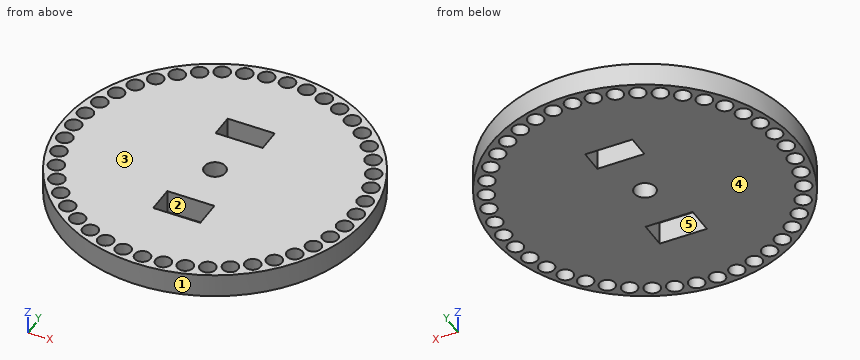
```python
from build123d import *

# Parameters (mm, degrees)
SKETCH1_R           = 19.5
BOSS_EXTRUDE1_DEPTH = 3
SKETCH6_R           = 1
CUT_EXTRUDE3_DEPTH  = 3
SKETCH7_R           = 1.35
CUT_EXTRUDE4_DEPTH  = 3
SKETCH10_W          = 6
SKETCH10_H          = 3
SKETCH10_H_2        = 3.5
CUT_EXTRUDE5_DEPTH  = 3


with BuildPart() as part:
    # Sketch1 → Boss-Extrude1 (new body)
    with BuildSketch(Plane.XY):
        Circle(SKETCH1_R)
    extrude(amount=BOSS_EXTRUDE1_DEPTH)

    # Sketch6 → Cut-Extrude3 (cut)
    with BuildSketch(Plane.XY.offset(3)):
        with Locations((0, 18)):
            Circle(SKETCH6_R)
        with Locations((2.561667089, 17.816785954)):
            Circle(SKETCH6_R)
        with Locations((5.071186023, 17.270873525)):
            Circle(SKETCH6_R)
        with Locations((7.477470234, 16.373375916)):
            Circle(SKETCH6_R)
        with Locations((9.731534714, 15.142563591)):
            Circle(SKETCH6_R)
        with Locations((11.787493211, 13.603492338)):
            Circle(SKETCH6_R)
        with Locations((13.603492338, 11.787493211)):
            Circle(SKETCH6_R)
        with Locations((15.142563591, 9.731534714)):
            Circle(SKETCH6_R)
        with Locations((16.373375916, 7.477470234)):
            Circle(SKETCH6_R)
        with Locations((17.270873525, 5.071186023)):
            Circle(SKETCH6_R)
        with Locations((17.816785954, 2.561667089)):
            Circle(SKETCH6_R)
        with Locations((18, 0)):
            Circle(SKETCH6_R)
        with Locations((17.816785954, -2.561667089)):
            Circle(SKETCH6_R)
        with Locations((17.270873525, -5.071186023)):
            Circle(SKETCH6_R)
        with Locations((16.373375916, -7.477470234)):
            Circle(SKETCH6_R)
        with Locations((15.142563591, -9.731534714)):
            Circle(SKETCH6_R)
        with Locations((13.603492338, -11.787493211)):
            Circle(SKETCH6_R)
        with Locations((11.787493211, -13.603492338)):
            Circle(SKETCH6_R)
        with Locations((9.731534714, -15.142563591)):
            Circle(SKETCH6_R)
        with Locations((7.477470234, -16.373375916)):
            Circle(SKETCH6_R)
        with Locations((5.071186023, -17.270873525)):
            Circle(SKETCH6_R)
        with Locations((2.561667089, -17.816785954)):
            Circle(SKETCH6_R)
        with Locations((0, -18)):
            Circle(SKETCH6_R)
        with Locations((-2.561667089, -17.816785954)):
            Circle(SKETCH6_R)
        with Locations((-5.071186023, -17.270873525)):
            Circle(SKETCH6_R)
        with Locations((-7.477470234, -16.373375916)):
            Circle(SKETCH6_R)
        with Locations((-9.731534714, -15.142563591)):
            Circle(SKETCH6_R)
        with Locations((-11.787493211, -13.603492338)):
            Circle(SKETCH6_R)
        with Locations((-13.603492338, -11.787493211)):
            Circle(SKETCH6_R)
        with Locations((-15.142563591, -9.731534714)):
            Circle(SKETCH6_R)
        with Locations((-16.373375916, -7.477470234)):
            Circle(SKETCH6_R)
        with Locations((-17.270873525, -5.071186023)):
            Circle(SKETCH6_R)
        with Locations((-17.816785954, -2.561667089)):
            Circle(SKETCH6_R)
        with Locations((-18, 0)):
            Circle(SKETCH6_R)
        with Locations((-17.816785954, 2.561667089)):
            Circle(SKETCH6_R)
        with Locations((-17.270873525, 5.071186023)):
            Circle(SKETCH6_R)
        with Locations((-16.373375916, 7.477470234)):
            Circle(SKETCH6_R)
        with Locations((-15.142563591, 9.731534714)):
            Circle(SKETCH6_R)
        with Locations((-13.603492338, 11.787493211)):
            Circle(SKETCH6_R)
        with Locations((-11.787493211, 13.603492338)):
            Circle(SKETCH6_R)
        with Locations((-9.731534714, 15.142563591)):
            Circle(SKETCH6_R)
        with Locations((-7.477470234, 16.373375916)):
            Circle(SKETCH6_R)
        with Locations((-5.071186023, 17.270873525)):
            Circle(SKETCH6_R)
        with Locations((-2.561667089, 17.816785954)):
            Circle(SKETCH6_R)
    extrude(amount=-CUT_EXTRUDE3_DEPTH, mode=Mode.SUBTRACT)

    # Sketch7 → Cut-Extrude4 (cut)
    with BuildSketch(Plane.XY.offset(3)):
        Circle(SKETCH7_R)
    extrude(amount=-CUT_EXTRUDE4_DEPTH, mode=Mode.SUBTRACT)

    # Sketch10 → Cut-Extrude5 (cut)
    with BuildSketch(Plane.XY.offset(3)):
        with Locations((0, 7.5)):
            Rectangle(SKETCH10_W, SKETCH10_H)
        with Locations((0, -7.75)):
            Rectangle(SKETCH10_W, SKETCH10_H_2)
    extrude(amount=-CUT_EXTRUDE5_DEPTH, mode=Mode.SUBTRACT)


solid = part.part
```
Build history of the part. All positions in model axes, mm. Face numbers are marked on the shaded views. A direction names the side the tool comes from. Give positions to 0.01 mm unless a question says otherwise; leave off trailing zeros. Loops run counter-clockwise (first coordinate to the right, second up) from the corner with the lowest first, then second, coordinate; pieces in that order, holes last.
1) Band-saw the part on A-A on x = 0. List the corners of the cut face in (y, z).
Values follow:
outline: (-19.5, 0) - (-19, 0) - (-19, 3) - (-19.5, 3) - close; (-17, 0) - (-9.5, 0) - (-9.5, 3) - (-17, 3) - close; (-6, 0) - (-1.35, 0) - (-1.35, 3) - (-6, 3) - close; (1.35, 0) - (6, 0) - (6, 3) - (1.35, 3) - close; (9, 0) - (17, 0) - (17, 3) - (9, 3) - close; (19, 0) - (19.5, 0) - (19.5, 3) - (19, 3) - close
2) Two-plate mould, pull along X, no slides. Class the marked faces 1, 2 and 3: released by +X, released by -X, zero draft, split by the parting line, or undercut.
Values follow:
face 1: split by the parting line
face 2: undercut
face 3: zero draft
3) Band-saw the part on C-C on x = -10. List the corners of the cut face in (y, z).
Values follow:
outline: (-16.74, 0) - (-16.11, 0) - (-16.11, 3) - (-16.74, 3) - close; (-14.18, 0) - (14.18, 0) - (14.18, 3) - (-14.18, 3) - close; (16.11, 0) - (16.74, 0) - (16.74, 3) - (16.11, 3) - close
4) 3-axis set-ups, long thin cutter, end or side, ignore diameter. For the marked faces 4 and 5: which of +Z, -Z, +X, -X, +Y, -Y reach the whole face in a straight line?
Values follow:
face 4: -Z, +X, -X, +Y, -Y
face 5: +Z, -Z
5) Band-saw the part on D-D on x = 12. List the corners of the cut face in (y, z).
Values follow:
outline: (-15.37, 0) - (-14.58, 0) - (-14.58, 3) - (-15.37, 3) - close; (-12.63, 0) - (12.63, 0) - (12.63, 3) - (-12.63, 3) - close; (14.58, 0) - (15.37, 0) - (15.37, 3) - (14.58, 3) - close
6) Drop flat-ended pins along their axis: P1, Ø1.6, axis at x = 11.79, y = 13.6, coming from the -Z side; P2, Ø1.5, axis at y = -4, z = 1.5, coming from the +X side; P3, Ø1.5, axis at y = 4.5, z = 0.5, coming from the -X side; P4, Ø0.9, axis at y = 7.5, z = 2, coming from the -X side. Give the stop position or say it passes through.
Values follow:
P1: passes through
P2: stops at x = 19.23
P3: stops at x = -19.14
P4: stops at x = -18.18
7) Band-saw the part on B-B on y = 0. List the corners of the cut face in (x, z), then the cut area to 3 significant figures.
Values follow:
outline: (-19.5, 0) - (-19, 0) - (-19, 3) - (-19.5, 3) - close; (-17, 0) - (-1.35, 0) - (-1.35, 3) - (-17, 3) - close; (1.35, 0) - (17, 0) - (17, 3) - (1.35, 3) - close; (19, 0) - (19.5, 0) - (19.5, 3) - (19, 3) - close
area: 96.9 mm2
8) Probe line 1 along Y through (x, z) = (9.5, 0.55); line 2 along X through (y, z) = (13.5, 2.7); line 3 along X through (y, z) = (-10, 0.6). List the from-to ranges inside material, lowest first.
Values follow:
line 1: y = -17.03 to -16.12, -14.17 to 14.17, 16.12 to 17.03
line 2: x = -14.07 to -12.78, -10.79 to 10.79, 12.78 to 14.07
line 3: x = -16.74 to -16.11, -14.18 to 14.18, 16.11 to 16.74
